Model file for the job. Use its own axes, mm. Face numbers are marked on the shaded views. A direction names the side the tool comes from. Round coordinates to 2 decimals unless told otherwise and drop trailing zeros. Order: outer loops, then holes, each group sorted by start corner. A loop starts at its lowest first (then second) coordinate and runs counter-clockwise, first axis right, second up. Notation, with made-up numbers: (85.5, -31.5) - (144.5, -31.5) arc R27 cw to (144.5, -7.5) - close; hole circle Ø11 at (40, 14.25). An arc over 180 degrees is marked (long way). Put each result on its own line as item: value. Start each with the question number.
Item 1: Saw through at C-C on x = 0.5. List the corners of the cut face in (y, z).
Item 2: Saw through at D-D on x = 2.5. List the corners of the cut face in (y, z).
Item 3: Saw through at B-B on z = 1.15. List the corners of the cut face in (x, y).
Item 4: Which spindle directions (+Z, -Z, +X, -X, +Y, -Y) get a long thin tool onto all of the face, cutting with end or side? Do the marked faces 4, 5 and 6. Say none if no direction does.
Item 5: Probe probe 1 along Y at (x, z) = (5.5, 2.3); probe 2 along X at (y, z) = (5, 1.85); probe 3 along X at (y, z) = (29.5, 2.5). List the from-to ranges inside material, lowest first.
Item 6: Mould opens along X. For the marked faces 1, 2 and 3 say: pulls with the +X half, pulls with the -X half, needs draft (parallel to the pull), parting line crosses it, or undercut.
Item 7: Pin check, flat tips, straight feed: pin 1 Ø0.6 at (x, z) = (10, 1.5) entering from -Y; pin 2 Ø0.9 at (y, z) = (25, 1) entering from -X; pin 3 Ø1.5 at (y, z) = (26.5, 1) entering from +X. Stop position of each tip, or through.
Item 8: Saw through at A-A on x = 5.5. List the corners of the cut face in (y, z), plus the area to 3 significant figures.
Autodesk Inventor part; units mm, degrees
ref_plane "YZ Plane" through (0, 0, 0) normal (1, 0, 0) x (0, 1, 0)
ref_plane "XZ Plane" through (0, 0, 0) normal (0, 1, 0) x (-1, 0, 0)
ref_plane "XY Plane" through (0, 0, 0) normal (0, 0, 1) x (1, 0, 0)
sketch "Sketch6" plane through (0, 0, 0) normal (0, 0, 1) x (1, 0, 0)
  line L0 (11, 34.8851) -> (0, 34.8851)
  line L1 (2, 31.8851) -> (2, 21.3851)
  line L2 (9, 31.8851) -> (9, 21.3851)
  line L3 (2, 21.3851) -> (0, 21.3851)
  line L4 (9, 21.3851) -> (11, 21.3851)
  arc A0 (0, 5.5) -> (11, 5.5) centre (5.5, 5.5) ccw
  circle A1 centre (5.5, 5.5) radius 1.5
  line L5 (0, 31.8851) -> (2, 31.8851)
  line L6 (9, 31.8851) -> (11, 31.8851)
  line L7 (0, 34.8851) -> (0, 31.8851)
  line L8 (0, 21.3851) -> (0, 5.5)
  line L9 (11, 5.5) -> (11, 21.3851)
  line L10 (11, 31.8851) -> (11, 34.8851)
  point P0 (0, 0)
  point P1 (10, 21.3851)
  dimension "d92" = 10.5
  dimension "d93" = 10.5
  dimension "d94" = 2
  dimension "d95" = 2
  dimension "d96" = 3
  dimension "d97" = 11
  dimension "d98" = 15.8851
extrude "Extrusion3" add sketch "Sketch6" along normal blind 3
properties part number "4P.01.01.16-BC-v1-Final Flap L2 80deg" material "Acrylic, Clear"
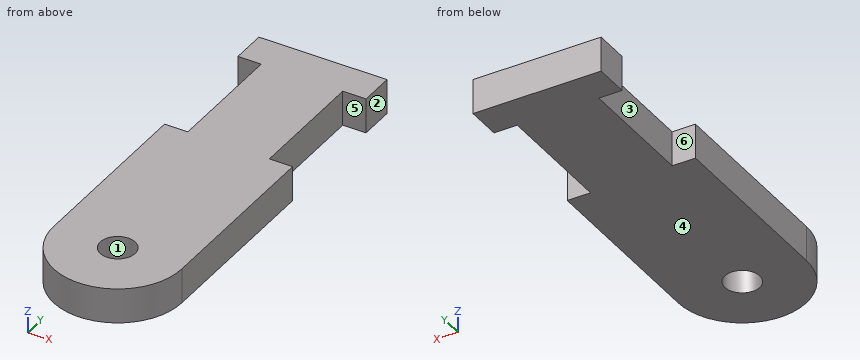
Results found:
1. outline: (3.21, 0) - (21.39, 0) - (21.39, 3) - (3.21, 3) - close; (31.89, 0) - (34.89, 0) - (34.89, 3) - (31.89, 3) - close
2. outline: (0.89, 0) - (34.89, 0) - (34.89, 3) - (0.89, 3) - close
3. outline: (0, 5.5) arc R5.5 ccw to (11, 5.5) - (11, 21.39) - (9, 21.39) - (9, 31.89) - (11, 31.89) - (11, 34.89) - (0, 34.89) - (0, 31.89) - (2, 31.89) - (2, 21.39) - (0, 21.39) - close; hole circle Ø3 at (5.5, 5.5)
4. face 4: -Z, +X, -X, +Y, -Y
4. face 5: +Z, -Z, +X
4. face 6: +Z, -Z, -X
5. probe 1: y = 0 to 4, 7 to 34.89
5. probe 2: x = 0.02 to 4.09, 6.91 to 10.98
5. probe 3: x = 2 to 9
6. face 1: undercut
6. face 2: pulls with the +X half
6. face 3: pulls with the -X half
7. pin 1: stops at y = 1.95
7. pin 2: stops at x = 2
7. pin 3: stops at x = 9
8. outline: (0, 0) - (4, 0) - (4, 3) - (0, 3) - close; (7, 0) - (34.89, 0) - (34.89, 3) - (7, 3) - close
8. area: 95.7 mm²
